Source: CAD feature listing. Evaluate the final solid. Frame: model axes, mm. Round coordinates to 2 decimals unless told otherwise and drop trailing zeros. Loops run counter-clockwise (first coordinate to the right, second up) from the corner with the lowest first, then second, coordinate; pieces in that order, holes last. Notation, with made-up numbers: M 30,44.5 L 85,44.5 A31 ccw 85,82.5 Z; hole C -34.5,40 d2. An arc over 180 degrees is marked long. Answer as a JSON object with one key per item and string values.
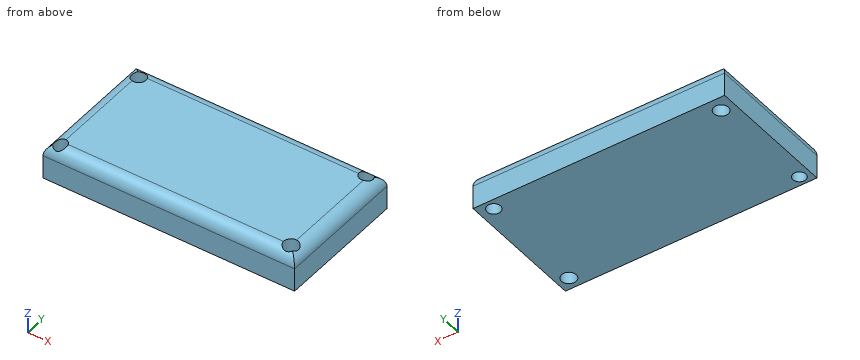
from build123d import *

# Parameters (mm, degrees)
F0_W        = 106.775932014
F0_H        = 55.2587080747
F0_R        = 2.7303671047
F0_R_2      = 3.1130972935
F0_R_3      = 3.09976381
F0_R_4      = 2.8780568391
F1_DEPTH    = 15
F2_T1_DEPTH = 131.775932014
F2_T3_DEPTH = 80.2587080747


# Not quite as in the source:
# - a fillet or chamfer that OpenCascade refuses, or shapes differently, is made with other operations: its cross-section is extruded or revolved along the edge and cut away or added


with BuildPart() as f1:
    # F0 (on Top) → F1 (new body)
    with BuildSketch(Plane.XY):
        with Locations((6.0439184308, 7.6268529519)):
            Rectangle(F0_W, F0_H)
        with Locations((-42.7391566336, -15.973219648)):
            Circle(F0_R, mode=Mode.SUBTRACT)
        with Locations((54.2513802648, -14.8219969124)):
            Circle(F0_R_2, mode=Mode.SUBTRACT)
        with Locations((-41.587933898, 29.2122848332)):
            Circle(F0_R_3, mode=Mode.SUBTRACT)
        with Locations((53.6757707596, 30.9391189367)):
            Circle(F0_R_4, mode=Mode.SUBTRACT)
    extrude(amount=F1_DEPTH)

    # F2: fillet of radius 5 on 4 edges, made by hand

    # F2_s2 → F2_t1 (cut)
    with BuildSketch(Plane.YZ.offset(-59.8440475762)):
        with BuildLine():
            ThreePointArc((-20.0025010854, 10), (-18.5380349913, 13.5355339059), (-15.0025010854, 15))
            Line((-15.0025010854, 15), (-20.0025010854, 15))
            Line((-20.0025010854, 15), (-20.0025010854, 10))
        make_face()
        with BuildLine():
            ThreePointArc((35.2562069893, 10), (33.7917408952, 13.5355339059), (30.2562069893, 15))
            Line((30.2562069893, 15), (35.2562069893, 15))
            Line((35.2562069893, 15), (35.2562069893, 10))
        make_face()
    extrude(amount=F2_T1_DEPTH, mode=Mode.SUBTRACT)

    # F2_s4 → F2_t3 (cut)
    with BuildSketch(Plane.XZ.offset(-47.7562069893)):
        with BuildLine():
            ThreePointArc((59.4318844378, 10), (57.9674183437, 13.5355339059), (54.4318844378, 15))
            Line((54.4318844378, 15), (59.4318844378, 15))
            Line((59.4318844378, 15), (59.4318844378, 10))
        make_face()
        with BuildLine():
            ThreePointArc((-47.3440475762, 10), (-45.8795814821, 13.5355339059), (-42.3440475762, 15))
            Line((-42.3440475762, 15), (-47.3440475762, 15))
            Line((-47.3440475762, 15), (-47.3440475762, 10))
        make_face()
    extrude(amount=F2_T3_DEPTH, mode=Mode.SUBTRACT)


solid = f1.part
Item 1: Section A-A on z = 12.75. Return the cut outline in (x, y).
Answer sheet:
{"outline": "M -46.52,-19.18 L 58.61,-19.18 L 58.61,34.43 L -46.52,34.43 Z; hole C -42.74,-15.97 d5.46; hole C -41.59,29.21 d6.2; hole C 53.68,30.94 d5.76; hole C 54.25,-14.82 d6.23"}
Item 2: Section B-B on z = 3.25. Return the cut outline in (x, y), then the cut area to 3 significant figures.
Answer sheet:
{"outline": "M -47.34,-20 L 59.43,-20 L 59.43,35.26 L -47.34,35.26 Z; hole C -42.74,-15.97 d5.46; hole C -41.59,29.21 d6.2; hole C 53.68,30.94 d5.76; hole C 54.25,-14.82 d6.23", "area": "5,790 mm²"}
Item 3: Line query: probe 1 along X at (y, z) = (-15, 12); probe 2 along X at (y, z) = (-14, 13.25); probe 3 along Y at (x, z) = (32, 10.5). Output: solid intervals per line, ascending. Write a range as from..to.
Answer sheet:
{"probe 1": "x = -46.93..-45.29, -40.19..51.14, 57.36..59.01", "probe 2": "x = -46.14..-44.63, -40.85..51.25, 57.25..58.23", "probe 3": "y = -19.98..35.23"}
Item 4: Contact query for a flat-ended pin moving along its axis: pin 1 Ø1.5 at (x, z) = (15.5, 11.5) entering from -Y. Output: stop coordinate, or through.
Answer sheet:
{"pin 1": "stops at y = -19.95"}
